For this review, take the finished solid that the model builds, in its own axes (mm). A direction names the side the tool comes from. Give positions to 0.01 mm unless a question says otherwise; leave off trailing zeros. Order: outer loops, then holes, each group sorted by start corner. A loop starts at its lowest first (then second) coordinate and runs counter-clockwise, first axis right, second up.
Item 1: Consider section C-C (z = 89). Give the boundary of the cut face in (x, y), plus the area to 3 significant figures.
Item 2: Machinability: for faces 4 (the cylindrical face through (-0.75, 5.7, 59.16)), 5 (the flat face through (77.5, -1, 2)), 6 (the flat face through (5, -5, 7)), which of the approach directions +Z, -Z, +X, -X, +Y, -Y give a long, thin tool a straight path to every point of the face, cutting with its end or side? Answer none if there is none.
Item 3: Consider section A-A (x = -55.5). Give the boundary of the cut face in (y, z), plus the area to 3 significant figures.
Item 4: Consider section D-D (x = 35). Give the boundary of the cut face in (y, z).
Item 5: Consider section B-B (y = 0). Give the boundary of the cut face in (x, z), plus the area to 3 significant figures.
Item 6: The part is to be moulded in two halves that separate along Y. For faces 1 (the cylindrical face through (48.13, 79.76, 2.46)), 2 (the flat face through (-1, 90, 2)), 3 (the cylindrical face through (-0.879, 6.693, 65.174)), say which applies: released by +Y, released by -Y, zero draft, split by the parting line, or undercut.
Item 7: For probe 1 along Y at (x, z) = (55, 3); probe 2 along Z at (x, y) = (55, -30); probe 3 along Y at (x, z) = (0, 37), list the stretches that pass through material, from the lowest coordinate up.
Item 8: For P1, Ø0.8, axis at x = 0.5, y = -6, coming from the -Z side; P2, Ø0.7, axis at x = -2.5, z = 45, coming from the -Y side; P3, Ø0.6, axis at y = -5.5, z = 40, coming from the -X side; P4, Ø3, axis at x = 59.5, y = 25, coming from the +Z side, all flat-tipped, find the tip position at first contact; note any pin that passes through.
```python
from build123d import *

# Parameters (mm, degrees)
SKETCH1_W           = 155
SKETCH1_H           = 180
SKETCH1_R           = 10
SKETCH1_R_2         = 12.5
BOSS_EXTRUDE1_DEPTH = 5
SKETCH1_3_R         = 12.5
SKETCH1_3_R_2       = 6.75
BOSS_EXTRUDE2_DEPTH = 7
SKETCH1_4_R         = 6.75
SKETCH1_4_R_2       = 5.75
BOSS_EXTRUDE3_DEPTH = 125
SKETCH1_5_R         = 5.75
CUT_EXTRUDE1_DEPTH  = 120
SKETCH2_W           = 6
SKETCH2_H           = 3.022470888
CUT_EXTRUDE2_DEPTH  = 80


with BuildPart() as part:
    # Sketch1 → Boss-Extrude1 (new body)
    with BuildSketch(Plane.XY):
        Rectangle(SKETCH1_W, SKETCH1_H)
        with Locations((55.5, -73)):
            Circle(SKETCH1_R, mode=Mode.SUBTRACT)
        with Locations((-55.5, -73)):
            Circle(SKETCH1_R, mode=Mode.SUBTRACT)
        Circle(SKETCH1_R_2, mode=Mode.SUBTRACT)
        with Locations((55.5, 73)):
            Circle(SKETCH1_R, mode=Mode.SUBTRACT)
        with Locations((-55.5, 73)):
            Circle(SKETCH1_R, mode=Mode.SUBTRACT)
    extrude(amount=BOSS_EXTRUDE1_DEPTH)

    # Sketch1_3 → Boss-Extrude2 (add)
    with BuildSketch(Plane.XY):
        Circle(SKETCH1_3_R)
        Circle(SKETCH1_3_R_2, mode=Mode.SUBTRACT)
    extrude(amount=BOSS_EXTRUDE2_DEPTH)

    # Sketch1_4 → Boss-Extrude3 (add)
    # profile 1 of 2: a face of its own
    with BuildSketch(Plane.XY):
        Circle(SKETCH1_4_R)
        Circle(SKETCH1_4_R_2, mode=Mode.SUBTRACT)
    # profile 2 of 2: a face of its own
    with BuildSketch(Plane.XY):
        Circle(SKETCH1_4_R_2)
    extrude(amount=BOSS_EXTRUDE3_DEPTH)

    # Sketch1_5 → Cut-Extrude1 (cut)
    with BuildSketch(Plane.XY):
        Circle(SKETCH1_5_R)
    extrude(amount=CUT_EXTRUDE1_DEPTH, mode=Mode.SUBTRACT)

    # Sketch2 → Cut-Extrude2 (cut)
    with BuildSketch(Plane.XY.offset(15)):
        with Locations((0, -6.75)):
            Rectangle(SKETCH2_W, SKETCH2_H)
    extrude(amount=CUT_EXTRUDE2_DEPTH, mode=Mode.SUBTRACT)


solid = part.part
```
Resolved:
1. outline: (-3, -6.05) - (-3, -5.24) - (-2.37, -5.24) arc R5.75 cw (long way) to (2.37, -5.24) - (3, -5.24) - (3, -6.05) arc R6.75 ccw (long way) to start
1. area: 33.2 mm2
2. face 4: -Z
2. face 5: +Z, -Z, +X, +Y, -Y
2. face 6: +Z
3. outline: (-90, 0) - (-83, 0) - (-83, 5) - (-90, 5) - close; (-63, 0) - (63, 0) - (63, 5) - (-63, 5) - close; (83, 0) - (90, 0) - (90, 5) - (83, 5) - close
3. area: 700 mm2
4. outline: (-90, 0) - (90, 0) - (90, 5) - (-90, 5) - close
5. outline: (-77.5, 0) - (-5.75, 0) - (-5.75, 120) - (5.75, 120) - (5.75, 0) - (77.5, 0) - (77.5, 5) - (12.5, 5) - (12.5, 7) - (6.75, 7) - (6.75, 125) - (-6.75, 125) - (-6.75, 7) - (-12.5, 7) - (-12.5, 5) - (-77.5, 5) - close
5. area: 1,040 mm2
6. face 1: undercut
6. face 2: released by +Y
6. face 3: split by the parting line
7. probe 1: y = -90 to -82.99, -63.01 to 63.01, 82.99 to 90
7. probe 2: z = 0 to 5
7. probe 3: y = 5.75 to 6.75
8. P1: stops at z = 0
8. P2: stops at y = -5.24
8. P3: stops at x = -4.3
8. P4: stops at z = 5
